Input: part model. Units: mm. Frame: model coordinates. A direction names the side the tool comes from. Coordinates: 2 decimals unless noted, no trailing zeros. Write each loop counter-clockwise with the first axis right and the second up, starting at its lowest first coordinate (ties: lowest second). Pieces come first, ordered by that corner, then holes. Notation, with made-up numbers: M 15.5,18 L 61.5,18 A25 cw 61.5,49 Z; hole C 61.5,-14.5 d3. An arc over 180 degrees is marked long. Use CSV: the item, a comma, the result in double quotes.
```python
from build123d import *

# Parameters (mm, degrees)
SKETCH_1_W          = 20
SKETCH_1_H          = 7
EXTRUDE_1_DEPTH     = 7.8
SKETCH_2_R          = 1.75
CUT_EXTRUDE_1_DEPTH = 7.8
SKETCH_3_W          = 2
SKETCH_3_H          = 3
CUT_EXTRUDE_2_DEPTH = 7.8


with BuildPart() as part:
    # 草图1 → 凸台-拉伸1 (new body)
    with BuildSketch(Plane.XY):
        Rectangle(SKETCH_1_W, SKETCH_1_H)
    extrude(amount=EXTRUDE_1_DEPTH)

    # 草图2 → 切除-拉伸1 (cut)
    with BuildSketch(Plane.XY.offset(7.8)):
        with Locations((-4.965, 0.85)):
            Circle(SKETCH_2_R)
        with Locations((4.965, 0.85)):
            Circle(SKETCH_2_R)
    extrude(amount=-CUT_EXTRUDE_1_DEPTH, mode=Mode.SUBTRACT)

    # 草图3 → 切除-拉伸2 (cut)
    with BuildSketch(Plane.XY.offset(7.8)):
        with Locations((0, -2)):
            Rectangle(SKETCH_3_W, SKETCH_3_H)
    extrude(amount=-CUT_EXTRUDE_2_DEPTH, mode=Mode.SUBTRACT)


solid = part.part
```
1. Section A-A (y = 0.85). Return loops of the section in (x, z) (3 decimals), then the cut area to 3 significant figures.
Resolved:
outline,"M -10,0 L -6.715,0 L -6.715,7.8 L -10,7.8 Z; M -3.215,0 L 3.215,0 L 3.215,7.8 L -3.215,7.8 Z; M 6.715,0 L 10,0 L 10,7.8 L 6.715,7.8 Z"
area,"101 mm^2"
2. Material intervals for line 1 (X direction, y = 0.5, z = 6); line 2 (X direction, y = 1.5, z = 4); line 3 (X direction, y = -1, z = 2), sorted ascending. Write a range as [from, to].
Resolved:
line 1,"x = [-10, -6.68], [-3.25, 3.25], [6.68, 10]"
line 2,"x = [-10, -6.59], [-3.34, 3.34], [6.59, 10]"
line 3,"x = [-10, -1], [1, 10]"
3. Section C-C (x = -5). Return loops of the section in (y, z), then the cut area to 3 significant figures.
Resolved:
outline,"M -3.5,0 L -0.9,0 L -0.9,7.8 L -3.5,7.8 Z; M 2.6,0 L 3.5,0 L 3.5,7.8 L 2.6,7.8 Z"
area,"27.3 mm^2"
4. Access query for faces 1 (the flat face through (1, -2, 4)), 2 (the cylindrical face through (3.217, 0.927, 3.955)). Directions: +Z, -Z, +X, -X, +Y, -Y. A direction counts if a zero-diameter tool reaches every point of the face in a straight line with its end or side. Return the directions, or none.
Resolved:
face 1,"+Z, -Z, -Y"
face 2,"+Z, -Z"
5. Mould query, pull axis Y, two halves, no side actions, for faces 3 (the cylindrical face through (-3.35, 0.18, 3.95)), 4 (the flat face through (0, 0, 7.8)), 5 (the flat face through (0, 3.5, 4)). Classes: pulls with the +Y half, pulls with the -Y half, needs draft (parallel to the pull), parting line crosses it, or undercut.
Resolved:
face 3,"undercut"
face 4,"needs draft"
face 5,"pulls with the +Y half"
6. Section B-B (z = 7.25). Return loops of the section in (x, y) (3 decimals), then the cut area to 3 significant figures.
Resolved:
outline,"M -10,-3.5 L -1,-3.5 L -1,-0.5 L 1,-0.5 L 1,-3.5 L 10,-3.5 L 10,3.5 L -10,3.5 Z; hole C -4.965,0.85 d3.5; hole C 4.965,0.85 d3.5"
area,"115 mm^2"
